For this review, take the finished solid that the model builds, in its own axes (mm). A direction names the side the tool comes from. Round coordinates to 2 decimals unless told otherwise and drop trailing zeros. Loops run counter-clockwise (first coordinate to the right, second up) from the corner with the lowest first, then second, coordinate; pieces in that order, holes last. Notation, with made-up numbers: (37.5, 7) -> (84.5, 7) arc R22 cw to (84.5, 15) -> close; hole circle Ø11 at (14, -2). An arc over 180 degrees is marked (long way). Use one line per item in the form item = value. Start each with the question number.
from build123d import *
from build123d.topology import SkipClean

# Parameters (mm, degrees)
EXTRUDE_1_DEPTH      = 25
CUT_EXTRUDE_4_DEPTH  = 80.457942189
SKETCH_7_W           = 16.60831278
SKETCH_7_H           = 38.473598513
CUT_EXTRUDE_14_DEPTH = 80.457942189
SKETCH_8_W           = 5
SKETCH_8_H           = 30.968526609
EXTRUDE_2_DEPTH      = 25
SKETCH_9_W           = 2.765387297
SKETCH_9_H           = 65
EXTRUDE_3_DEPTH      = 100
SKETCH_10_W          = 5.026813651
SKETCH_10_H          = 30.968526609
EXTRUDE_4_DEPTH      = 40
CUT_EXTRUDE_15_DEPTH = 100
SKETCH_12_R          = 28.5
CUT_EXTRUDE_16_DEPTH = 100
SKETCH_13_R          = 1.25
CUT_EXTRUDE_17_DEPTH = 100
SKETCH_14_W          = 5.026813651
SKETCH_14_H          = 100.124810737
CUT_EXTRUDE_19_DEPTH = 165.009199789
SKETCH_15_W          = 2.026813651
SKETCH_15_H          = 30.843715872
CUT_EXTRUDE_20_DEPTH = 165.009199789
SKETCH_16_W          = 99.968526609
SKETCH_16_H          = 65
SKETCH_16_R          = 28.5
SKETCH_16_R_2        = 1.25
EXTRUDE_5_DEPTH      = 3
EXTRUDE_7_REACH      = 157.801
SKETCH_17_W          = 3.738573646
SKETCH_17_H          = 3
CHAMFER_1_DEPTH      = 25
SKETCH_18_W          = 3
SKETCH_18_H          = 64.869017051
EXTRUDE_8_DEPTH      = 2


with BuildPart() as part:
    # Эскиз1 → Бобышка-Вытянуть1 (new body)
    with BuildSketch(Plane(origin=(0, 0, 0), x_dir=(1, 0, 0), z_dir=(0, 1, 0))):
        Polygon((-66.825757576, 34.969739794), (-66.825757576, 29.969739794), (-63.825757576, 29.969739794), (-63.825757576, 31.969739794), (-38.825757576, 31.969739794), (-38.825757576, 6.969739794), (-63.825757576, 6.969739794), (-63.825757576, 8.969739794), (-66.825757576, 8.969739794), (-66.825757576, 3.969739794), (-22.123470102, 3.969739794), (-36.579007505, 34.969739794), align=None)
    extrude(amount=EXTRUDE_1_DEPTH)

    # Эскиз3 → Вырез-Вытянуть4 (cut, through all)
    with BuildSketch(Plane.XZ):
        Polygon((-66.825757576, -3.969739794), (-65.325757576, -8.969739794), (-66.825757576, -8.969739794), align=None)
        Polygon((-66.825757576, -29.969739794), (-66.825757576, -34.969739794), (-65.325757576, -29.969739794), align=None)
    extrude(amount=-CUT_EXTRUDE_4_DEPTH, mode=Mode.SUBTRACT)

    # Эскиз7 → Вырез-Вытянуть14 (cut, through all)
    with BuildSketch(Plane(origin=(0, 0, 0), x_dir=(-1, 0, 0), z_dir=(0, -1, 0))):
        with Locations((27.703474463, 20.539743139)):
            Rectangle(SKETCH_7_W, SKETCH_7_H)
    extrude(amount=-CUT_EXTRUDE_14_DEPTH, mode=Mode.SUBTRACT)

    # Эскиз8 → Бобышка-Вытянуть2 (add)
    with BuildSketch(Plane(origin=(0, 0, 0), x_dir=(-1, 0, 0), z_dir=(0, -1, 0))):
        with Locations((36.298943925, 19.454003098)):
            Rectangle(SKETCH_8_W, SKETCH_8_H)
    extrude(amount=-EXTRUDE_2_DEPTH)

    # Эскиз9 → Бобышка-Вытянуть3 (add)
    with BuildSketch(Plane(origin=(0, 0, -34.938266403), x_dir=(-1, 0, 0), z_dir=(0, 0, -1))):
        with Locations((38.181637573, 32.5)):
            Rectangle(SKETCH_9_W, SKETCH_9_H)
    extrude(amount=EXTRUDE_3_DEPTH)

    # Эскиз10 → Бобышка-Вытянуть4 (add)
    with BuildSketch(Plane(origin=(0, 25, 0), x_dir=(1, 0, 0), z_dir=(0, 1, 0))):
        with Locations((-36.312350751, 19.454003098)):
            Rectangle(SKETCH_10_W, SKETCH_10_H)
    extrude(amount=EXTRUDE_4_DEPTH)

    # Эскиз11 → Вырез-Вытянуть15 (cut)
    with BuildSketch(Plane(origin=(-33.798943925, 0, 0), x_dir=(0, 0, -1), z_dir=(1, 0, 0))):
        Polygon((34.938266403, 65), (3.969739794, 32.5), (3.969739794, 65), align=None)
    extrude(amount=-CUT_EXTRUDE_15_DEPTH, mode=Mode.SUBTRACT)

    # Эскиз12 → Вырез-Вытянуть16 (cut)
    with BuildSketch(Plane(origin=(-36.798943925, 0, 0), x_dir=(0, 0, -1), z_dir=(1, 0, 0))):
        with Locations((102.438266403, 32.5)):
            Circle(SKETCH_12_R)
    extrude(amount=-CUT_EXTRUDE_16_DEPTH, mode=Mode.SUBTRACT)

    # Эскиз13 → Вырез-Вытянуть17 (cut)
    with BuildSketch(Plane(origin=(-36.798943925, 0, 0), x_dir=(0, 0, -1), z_dir=(1, 0, 0))):
        with Locations((77.438266403, 57.5)):
            Circle(SKETCH_13_R)
        with Locations((127.438266403, 57.5)):
            Circle(SKETCH_13_R)
        with Locations((127.438266403, 7.5)):
            Circle(SKETCH_13_R)
        with Locations((77.438266403, 7.5)):
            Circle(SKETCH_13_R)
    extrude(amount=-CUT_EXTRUDE_17_DEPTH, mode=Mode.SUBTRACT)

    # Эскиз14 → Вырез-Вытянуть19 (cut, through all)
    with BuildSketch(Plane(origin=(0, 0, 0), x_dir=(-1, 0, 0), z_dir=(0, -1, 0))):
        with Locations((36.312350751, 84.875861035)):
            Rectangle(SKETCH_14_W, SKETCH_14_H)
    extrude(amount=-CUT_EXTRUDE_19_DEPTH, mode=Mode.SUBTRACT)

    # Эскиз15 → Вырез-Вытянуть20 (cut, through all)
    with BuildSketch(Plane.XZ):
        with Locations((-34.812350751, -19.39159773)):
            Rectangle(SKETCH_15_W, SKETCH_15_H)
    extrude(amount=-CUT_EXTRUDE_20_DEPTH, mode=Mode.SUBTRACT)

    # Эскиз16 → Бобышка-Вытянуть5 (add)
    with SkipClean():  # the faces are left unmerged after this step: merging them gives an invalid solid
        with BuildSketch(Plane.ZY.offset(39.564331222)):
            with Locations((-84.954003098, 32.5)):
                Rectangle(SKETCH_16_W, SKETCH_16_H)
            with Locations((-102.438266403, 32.5)):
                Circle(SKETCH_16_R, mode=Mode.SUBTRACT)
            with Locations((-127.438266403, 57.5)):
                Circle(SKETCH_16_R_2, mode=Mode.SUBTRACT)
            with Locations((-77.438266403, 57.5)):
                Circle(SKETCH_16_R_2, mode=Mode.SUBTRACT)
            with Locations((-77.438266403, 7.5)):
                Circle(SKETCH_16_R_2, mode=Mode.SUBTRACT)
            with Locations((-127.438266403, 7.5)):
                Circle(SKETCH_16_R_2, mode=Mode.SUBTRACT)
        extrude(amount=EXTRUDE_5_DEPTH)

    # Бобышка-Вытянуть7: up to this plane
    with SkipClean():  # the faces are left unmerged after this step: merging them gives an invalid solid
        extrude_7_end = Plane(origin=(-133.798943925, 65, -34.938266403), z_dir=(0, -0.6898437432956686, -0.7239582928842101))
        # Эскиз17 → Бобышка-Вытянуть7 (add, up to the surface)
        with BuildSketch(Plane(origin=(0, 25, 0), x_dir=(1, 0, 0), z_dir=(0, 1, 0)), mode=Mode.PRIVATE) as extrude_7_sk1:
            with Locations((-40.695044399, 33.469739794)):
                Rectangle(SKETCH_17_W, SKETCH_17_H)
        extrude_7_tool1 = split(extrude(extrude_7_sk1.sketch, amount=EXTRUDE_7_REACH, mode=Mode.PRIVATE), bisect_by=extrude_7_end, keep=Keep.BOTH, mode=Mode.PRIVATE)
        add(extrude_7_tool1.solids().sort_by_distance((-40.695044, 25, -33.46974))[0])

    # Фаска1: read off the stored shape, not the designer's step
    # Фаска1 outline → Фаска1 (add)
    with SkipClean():  # the faces are left unmerged after this step: merging them gives an invalid solid
        with BuildSketch(Plane(origin=(0, 0, 0), x_dir=(1, 0, 0), z_dir=(0, 1, 0))):
            Polygon((-42.564331222, 44.969739794), (-52.564331222, 34.969739794), (-42.564331222, 34.969739794), align=None)
        extrude(amount=CHAMFER_1_DEPTH)

    # Эскиз18 → Бобышка-Вытянуть8 (add)
    with SkipClean():  # the faces are left unmerged after this step: merging them gives an invalid solid
        with BuildSketch(Plane(origin=(0, 0, -34.813455666), x_dir=(-1, 0, 0), z_dir=(0, 0, -1))):
            with Locations((37.325757576, 32.434508526)):
                Rectangle(SKETCH_18_W, SKETCH_18_H)
        extrude(amount=EXTRUDE_8_DEPTH)


solid = part.part
Item 1: Take a section at A-A on x = -57. Give the boundary of the cut face in (y, z).
Item 2: For P1, Ø3, axis at y = 7.5, z = -127.44, coming from the +X side; P2, Ø2, axis at y = 57.5, z = -127.44, coming from the -X side; P3, Ø1, axis at y = 58, z = -37.5, coming from the -X side; P4, Ø12, axis at x = -42, z = -118.5, coming from the +Y side, all flat-tipped, find the tip position at first contact; note any pin that passes through.
Item 3: Wall thickness on line 1 (Z direction, x = -41, y = 32); line 2 (X direction, y = 3, z = -31); line 3 (Z direction, x = -38.5, y = 3): over which ranges is each line inside the solid? List them lowest first.
Item 4: Take a section at B-B on y = 7.5. Give the number of separate pieces and of enclosed holes in the cut face, plus the area to 3 significant figures.
Item 5: Take a section at D-D on y = 52.5. Give the boundary of the cut face in (x, z), plus the area to 3 significant figures.
Item 6: Take a section at C-C on z = -118. Give the boundary of the cut face in (x, y), plus the area to 3 significant figures.
Item 7: Machinability: for faces 1 (the flat face through (-66.086, 12.325, -32.505)), 2 (the flat face through (-52, 12, -3.97)), 3 (the flat face through (-37, 33, -36.813)), which of the approach directions +Z, -Z, +X, -X, +Y, -Y give a long, thin tool a straight path to every point of the face, cutting with its end or side? Answer none if there is none.
Item 8: Draft analysis for pull direction Z (two halves, no side actions). For faces 4 (the flat face through (-60, 12, -34.97)), 5 (the flat face through (-53, 25, -5)), 6 (the flat face through (-51, 12, -6.97)), state which applies: +Z half, -Z half, draft (parallel to the pull), parting line (faces both ways), or undercut.
Results:
q1.outline = (0, -34.97) -> (25, -34.97) -> (25, -31.97) -> (0, -31.97) -> close; (0, -6.97) -> (25, -6.97) -> (25, -3.97) -> (0, -3.97) -> close
q2.P1 = -38.83
q2.P2 = through
q2.P3 = -42.56
q2.P4 = 65
q3.line_1 = -134.94 to -130.93, -73.94 to -31.97
q3.line_2 = -65.63 to -63.83, -38.83 to -35.83
q3.line_3 = -36.81 to -3.97
q4.separate_pieces = 4
q4.enclosed_holes = 0
q4.area = 574 mm2
q5.outline = (-42.56, -134.94) -> (-38.83, -134.94) -> (-38.83, -122.74) -> (-42.56, -122.74) -> close; (-42.56, -82.13) -> (-38.83, -82.13) -> (-38.83, -36.81) -> (-35.83, -36.81) -> (-35.83, -23.03) -> (-38.83, -23.03) -> (-38.83, -31.97) -> (-42.56, -31.97) -> close
q5.area = 274 mm2
q6.outline = (-42.56, 0) -> (-38.83, 0) -> (-38.83, 8.62) -> (-42.56, 8.62) -> close; (-42.56, 56.38) -> (-38.83, 56.38) -> (-38.83, 65) -> (-42.56, 65) -> close
q6.area = 64.5 mm2
q7.face_1 = -X, +Y, -Y
q7.face_2 = +Z, +X, -X, +Y, -Y
q7.face_3 = -Z, +X, +Y, -Y
q8.face_4 = -Z half
q8.face_5 = draft
q8.face_6 = undercut
